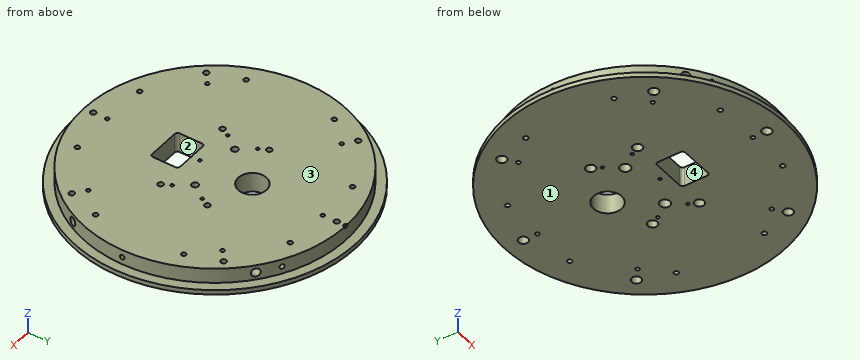
from build123d import *

# Parameters (mm, degrees)
SKETCH_1_R                   = 150
EXTRUDE_1_DEPTH              = 5
SKETCH_2_R                   = 140
EXTRUDE_2_DEPTH              = 16
SKETCH_3_R                   = 15
SKETCH_3_W                   = 40
SKETCH_3_H                   = 30
CUT_EXTRUDE_1_DEPTH          = 214.168947082
FILLET_2_R                   = 3
HOLE_WIZARD_M5_1_D           = 5.8
HOLE_WIZARD_M5_1_CBORE_D     = 10
HOLE_WIZARD_M5_1_CBORE_DEPTH = 8
HOLE_WIZARD_M6_1_D           = 7
HOLE_WIZARD_M6_1_CBORE_D     = 11
HOLE_WIZARD_M6_1_CBORE_DEPTH = 9
HOLE_WIZARD_M5_2_D           = 5.8
HOLE_WIZARD_M5_2_CBORE_D     = 10
HOLE_WIZARD_M5_2_CBORE_DEPTH = 8
M4X0_7_1_D                   = 3.3
M6X1_0_1_D                   = 5
PATTERN_CIRCULAR_1_COUNT     = 8
SKETCH_14_R                  = 2.5
CUT_EXTRUDE_2_DEPTH          = 2
M5X0_8_1_D                   = 4.2
PATTERN_CIRCULAR_2_COUNT     = 6
M10X1_0_1_D                  = 9
M10X1_0_1_DEPTH              = 25
M10X1_0_1_TIP                = 2.703872786
M10X1_0_1_ON_FACE_2_D        = 9
M10X1_0_1_ON_FACE_2_DEPTH    = 25
M10X1_0_1_ON_FACE_2_TIP      = 2.703872786
M10X1_0_1_ON_FACE_3_D        = 9
M10X1_0_1_ON_FACE_3_DEPTH    = 25
M10X1_0_1_ON_FACE_3_TIP      = 2.703872786
M10X1_0_1_ON_FACE_4_D        = 9
M10X1_0_1_ON_FACE_4_DEPTH    = 25
M10X1_0_1_ON_FACE_4_TIP      = 2.703872786


with BuildPart() as part:
    # ｽｹｯﾁ1 → ﾎﾞｽ - 押し出し1 (new body)
    with BuildSketch(Plane.XY):
        Circle(SKETCH_1_R)
    extrude(amount=EXTRUDE_1_DEPTH)

    # ｽｹｯﾁ2 → ﾎﾞｽ - 押し出し2 (add)
    with BuildSketch(Plane.XY.offset(5)):
        Circle(SKETCH_2_R)
    extrude(amount=EXTRUDE_2_DEPTH)

    # ｽｹｯﾁ3 → ｶｯﾄ - 押し出し1 (cut, through all)
    with BuildSketch(Plane(origin=(0, 0, 0), x_dir=(-1, 0, 0), z_dir=(0, 0, -1))):
        with Locations((0, 40)):
            Circle(SKETCH_3_R)
        with Locations((0, -40)):
            Rectangle(SKETCH_3_W, SKETCH_3_H)
    extrude(amount=-CUT_EXTRUDE_1_DEPTH, mode=Mode.SUBTRACT)

    # ﾌｨﾚｯﾄ2
    fillet_2_edges = [part.edges().sort_by_distance(p)[0] for p in [
        (-20, -25, 10.5),
        (-20, -55, 10.5),
        (20, -55, 10.5),
        (20, -25, 10.5),
    ]]
    fillet(fillet_2_edges, radius=FILLET_2_R)

    # M5 穴付きねじ用座ぐり穴1 (through all)
    with Locations(Plane(origin=(0, 130, 0), x_dir=(-1, 0, 0), z_dir=(0, 0, -1))):
        with Locations((0, 0), (101.640113623, -48.948859954), (-101.640113623, -48.948859954), (-101.640113623, -211.051140046), (0, -260), (101.640113623, -211.051140046)):
            CounterBoreHole(HOLE_WIZARD_M5_1_D / 2, HOLE_WIZARD_M5_1_CBORE_D / 2, HOLE_WIZARD_M5_1_CBORE_DEPTH)

    # M6 穴付きねじ用座ぐり穴1 (through all)
    with Locations(Plane(origin=(30, 0, 0), x_dir=(-1, 0, 0), z_dir=(0, 0, -1))):
        with Locations((0, 0), (60, 0)):
            CounterBoreHole(HOLE_WIZARD_M6_1_D / 2, HOLE_WIZARD_M6_1_CBORE_D / 2, HOLE_WIZARD_M6_1_CBORE_DEPTH)

    # M5 穴付きねじ用座ぐり穴2 (through all)
    with Locations(Plane(origin=(46.733285782, 25, 0), x_dir=(-1, 0, 0), z_dir=(0, 0, -1))):
        with Locations((0, 0), (0, -50), (93.466571564, 0), (93.466571564, -50)):
            CounterBoreHole(HOLE_WIZARD_M5_2_D / 2, HOLE_WIZARD_M5_2_CBORE_D / 2, HOLE_WIZARD_M5_2_CBORE_DEPTH)

    # M4x0.7 ねじ穴1 (through all)
    with Locations(Plane(origin=(42, 16, 0), x_dir=(-1, 0, 0), z_dir=(0, 0, -1))):
        with Locations((0, 0), (84, 0), (84, -32), (42, -32), (0, -32)):
            Hole(M4X0_7_1_D / 2)

    # M6x1.0 ねじ穴1 (through all)
    with Locations(Plane(origin=(-113.637182499, 47.070062181, 0), x_dir=(-1, 0, 0), z_dir=(0, 0, -1))):
        with Locations((0, 0)):
            m6x1_0_1 = Hole(M6X1_0_1_D / 2)

    # 円形ﾊﾟﾀｰﾝ1: M6x1.0 ねじ穴1 ×8 about axis
    pattern_circular_1_axis = Axis((0, 0, 0), (0, 0, 1))
    for i in range(1, PATTERN_CIRCULAR_1_COUNT):
        add(m6x1_0_1.rotate(pattern_circular_1_axis, i * 360 / PATTERN_CIRCULAR_1_COUNT), mode=Mode.SUBTRACT)

    # ｽｹｯﾁ14 → ｶｯﾄ - 押し出し2 (cut)
    with BuildSketch(Plane(origin=(0, 0, 21), x_dir=(-1, 0, 0), z_dir=(0, 0, -1))):
        with Locations((0, 140)):
            Circle(SKETCH_14_R)
    extrude(amount=CUT_EXTRUDE_2_DEPTH, mode=Mode.SUBTRACT)

    # M5x0.8 ねじ穴1 (through all)
    with Locations(Plane(origin=(-89.912408205, 71.699085425, 0), x_dir=(-1, 0, 0), z_dir=(0, 0, -1))):
        with Locations((0, 0), (0, -143.39817085), (-89.912408205, -186.699085425), (-179.82481641, -143.39817085), (-179.82481641, 0), (-89.912408205, 43.300914575)):
            Hole(M5X0_8_1_D / 2)

    # ｽｹｯﾁ19 → M6x1.0 ねじ穴2 (revolve, cut)
    with BuildSketch(Plane(origin=(140, 0, 13), x_dir=(0, 0, -1), z_dir=(0, 1, 0))):
        Polygon((0, 0), (0, 21.502151548), (2.5, 20), (2.5, 0), align=None)
    m6x1_0_2 = revolve(axis=Axis((146.35, 0, 13), (-1, 0, 0)), mode=Mode.SUBTRACT)

    # 円形ﾊﾟﾀｰﾝ2: M6x1.0 ねじ穴2 ×6 about axis
    pattern_circular_2_axis = Axis((0, 0, -1.05), (0, 0, 1))
    for i in range(1, PATTERN_CIRCULAR_2_COUNT):
        add(m6x1_0_2.rotate(pattern_circular_2_axis, i * 360 / PATTERN_CIRCULAR_2_COUNT), mode=Mode.SUBTRACT)

    # M10x1.0 ねじ穴1
    with Locations(Plane(origin=(-89.990265356, 107.246222037, 13), x_dir=(0.766044443119, 0.642787609687, 0), z_dir=(-0.642787609687, 0.766044443119, 0))):
        with Locations((0, 0)):
            Hole(M10X1_0_1_D / 2, depth=M10X1_0_1_DEPTH)
            with Locations((0, 0, -(M10X1_0_1_DEPTH + M10X1_0_1_TIP / 2))):  # 118° drill point
                Cone(0, M10X1_0_1_D / 2, M10X1_0_1_TIP, mode=Mode.SUBTRACT)

    # M10x1.0 ねじ穴1 on face 2
    with Locations(Plane(origin=(89.990265356, 107.246222037, 13), x_dir=(0.766044067841, -0.642788056925, 0), z_dir=(0.642788056925, 0.766044067841, 0))):
        with Locations((0, 0)):
            Hole(M10X1_0_1_ON_FACE_2_D / 2, depth=M10X1_0_1_ON_FACE_2_DEPTH)
            with Locations((0, 0, -(M10X1_0_1_ON_FACE_2_DEPTH + M10X1_0_1_ON_FACE_2_TIP / 2))):  # 118° drill point
                Cone(0, M10X1_0_1_ON_FACE_2_D / 2, M10X1_0_1_ON_FACE_2_TIP, mode=Mode.SUBTRACT)

    # M10x1.0 ねじ穴1 on face 3
    with Locations(Plane(origin=(124.740913386, -63.558669964, 13), x_dir=(0.45398991053, 0.891006824405, 0), z_dir=(0.891006824405, -0.45398991053, 0))):
        with Locations((1e-09, 0)):
            Hole(M10X1_0_1_ON_FACE_3_D / 2, depth=M10X1_0_1_ON_FACE_3_DEPTH)
            with Locations((0, 0, -(M10X1_0_1_ON_FACE_3_DEPTH + M10X1_0_1_ON_FACE_3_TIP / 2))):  # 118° drill point
                Cone(0, M10X1_0_1_ON_FACE_3_D / 2, M10X1_0_1_ON_FACE_3_TIP, mode=Mode.SUBTRACT)

    # M10x1.0 ねじ穴1 on face 4
    with Locations(Plane(origin=(-89.990265356, -107.246222037, 13), x_dir=(-0.766044067841, 0.642788056925, 0), z_dir=(-0.642788056925, -0.766044067841, 0))):
        with Locations((0, 0)):
            Hole(M10X1_0_1_ON_FACE_4_D / 2, depth=M10X1_0_1_ON_FACE_4_DEPTH)
            with Locations((0, 0, -(M10X1_0_1_ON_FACE_4_DEPTH + M10X1_0_1_ON_FACE_4_TIP / 2))):  # 118° drill point
                Cone(0, M10X1_0_1_ON_FACE_4_D / 2, M10X1_0_1_ON_FACE_4_TIP, mode=Mode.SUBTRACT)


solid = part.part
Input: part model. Units: mm. Frame: model coordinates. Face numbers are marked on the shaded views. A direction names the side the tool comes from. Coordinates: 2 decimals unless noted, no trailing zeros. Answer in a Markdown table with one row per item. Add a question column.
Item 1: Line query: line 1 along Y through (x, z) = (90.5, 13.75); line 2 along X through (y, z) = (-130, 14.75); line 3 along X through (y, z) = (-54.5, 2). Output: solid intervals per line, ascending. Write a range as [from, to].
Item 2: Mould query, pull axis Y, two halves, no side actions, for the marked faces 1 and 2. Classes: released by +Y, released by -Y, zero draft, split by the parting line, or undercut.
Item 3: Contact query for flat-ended pins moving along their axis: P1, Ø1, axis at x = -89, z = 8, coming from the -Y side; P2, Ø5, axis at x = 47.5, y = -24, coming from the -Z side; P3, Ø8, axis at x = -15, z = 16.5, coming from the +Y side. Output: stop coordinate, or through.
Item 4: Access query for the marked faces 3 and 4. Directions: +Z, -Z, +X, -X, +Y, -Y. A direction counts if a zero-diameter tool reaches every point of the face in a straight line with its end or side. Return the directions, or none.
Recorded:
| question | item | result |
|---|---|---|
| 1 | line 1 | [-106.82, -73.72], [-69.68, 69.68], [73.72, 100.95] |
| 1 | line 2 | [-51.96, -2.9], [2.9, 51.96] |
| 1 | line 3 | [-139.75, -18.66], [18.66, 139.75] |
| 2 | face 1 | zero draft |
| 2 | face 2 | undercut |
| 3 | P1 | y = -108.48 |
| 3 | P2 | z = 8 |
| 3 | P3 | y = 139.57 |
| 4 | face 3 | +Z, +X, -X, +Y, -Y |
| 4 | face 4 | +Z, -Z |
